Check sheet for the drawn part. Datum: minimum x, y, z corner. Units: mm. Coordinates: 2 decimals unless noted, no trailing zeros. Order: outer loops, then holes, each group sorted by start corner. A loop starts at its lowest first (then second) coordinate and runs counter-clockwise, first axis right, second up. Notation, with made-up numbers: M 12.5,-2.75 L 71.5,-2.75 A23 ccw 71.5,23.25 Z; hole C 85.5,37 d10. An arc over 180 degrees is marked long. Use one line per item in the form item = value. Start each with the question number.
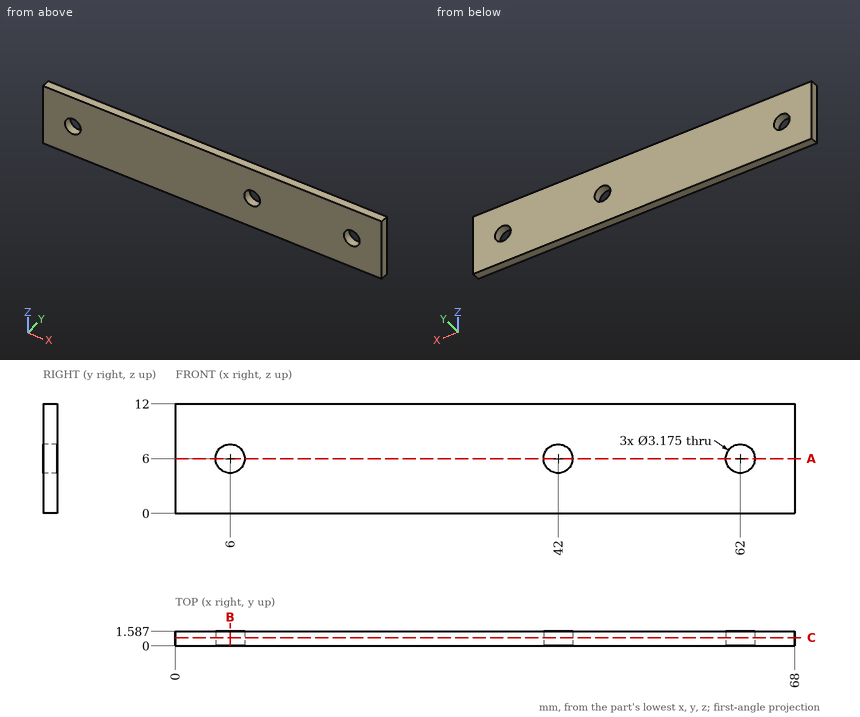
1. Cross-section at A-A on z = 6. Enter the section's corners in (x, y).
2. Cross-section at B-B on x = 6. Enter the section's corners in (y, z), and give its area (3 significant figures).
3. Depth check by flat-ended pin: P1, Ø3.5, axis at x = 42, z = 6, coming from the -Y side; P2, Ø3, axis at x = 62, z = 6, coming from the -Y side. Enter the tip coordinate at first touch or a pass-through.
4. Cross-section at C-C on y = 0.9. Enter the section's corners in (x, z) (1 decimal).
5. Material ranges on line 1 along X through (y, z) = (0.8, 6); line 2 along X through (y, z) = (1.05, 5) (1 decimal), recorded low to high.
Final values:
q1.outline = M 0,0 L 4.41,0 L 4.41,1.59 L 0,1.59 Z; M 7.59,0 L 40.41,0 L 40.41,1.59 L 7.59,1.59 Z; M 43.59,0 L 60.41,0 L 60.41,1.59 L 43.59,1.59 Z; M 63.59,0 L 68,0 L 68,1.59 L 63.59,1.59 Z
q2.outline = M 0,0 L 1.59,0 L 1.59,4.41 L 0,4.41 Z; M 0,7.59 L 1.59,7.59 L 1.59,12 L 0,12 Z
q2.area = 14.0 mm2
q3.P1 = 0
q3.P2 = through
q4.outline = M 0,0 L 68,0 L 68,12 L 0,12 Z; hole C 6,6 d3.2; hole C 42,6 d3.2; hole C 62,6 d3.2
q5.line_1 = 0 to 4.41, 7.59 to 40.41, 43.59 to 60.41, 63.59 to 68
q5.line_2 = 0 to 4.8, 7.2 to 40.8, 43.2 to 60.8, 63.2 to 68
